Part model, mm, in its own coordinate system. A direction names the side the tool comes from. Give positions to 0.01 mm unless a question says otherwise; leave off trailing zeros. Order: outer loops, then holes, each group sorted by start corner. A loop starts at its lowest first (then second) coordinate and runs counter-clockwise, first axis right, second up.
1. Mould opens along Z. For faces 3 (the flat face through (20, 3, -41)), 4 (the flat face through (39, 3, -2)), 5 (the flat face through (3, 3, -36)) say: +Z half, -Z half, draft (parallel to the pull), parting line (faces both ways), or undercut.
2. Drop flat-ended pins along their axis: pin 1 Ø1 at (x, z) = (5, -12.5) entering from -Y; pin 2 Ø3 at (y, z) = (-5.5, -36.5) entering from -X; pin 3 Ø3.5 at (x, z) = (21, -6) entering from -Y. Give the stop position or say it passes through.
3. Which spindle directions (+Z, -Z, +X, -X, +Y, -Y) get a long thin tool onto all of the face, cutting with end or side? Do faces 1 (the cylindrical face through (32, -20.54, -10.57)), 2 (the cylindrical face through (37.2, 4, -4.1)). Say none if no direction does.
4. Probe line 1 (Z direction, x = 5, y = 1.85); line 2 (X direction, y = -22, z = -19); line 3 (Z direction, x = 10.5, y = -21.2). List the from-to ranges inside material, lowest first.
5. Slice it at A-A on y = -20. Give the number of separate pieces and of enclosed holes in the cut face, and give its area (3 significant figures).
6. Slice it at B-B on y = -11.5. List the corners of the cut face in (x, z).
from build123d import *

# Parameters (mm, degrees)
SKETCH1_W           = 41
SKETCH1_H           = 41
BOSS_EXTRUDE1_DEPTH = 5
CUT_EXTRUDE2_DEPTH  = 5
SKETCH4_R           = 11.5
CUT_EXTRUDE3_DEPTH  = 2
SKETCH6_R           = 17.5
BOSS_EXTRUDE2_DEPTH = 23
FILLET1_R           = 0.2
FILLET2_R           = 0.5
SKETCH13_R          = 11
BOSS_EXTRUDE3_DEPTH = 2
SKETCH5_R           = 3
CUT_EXTRUDE9_DEPTH  = 31
SKETCH14_R          = 2.5
CUT_EXTRUDE10_DEPTH = 5
SKETCH15_R          = 1.5
CUT_EXTRUDE11_DEPTH = 5
SKETCH16_R          = 2.5
CUT_EXTRUDE12_DEPTH = 3
SKETCH17_R          = 1.5
CUT_EXTRUDE13_DEPTH = 3
SKETCH18_R          = 1.5
CUT_EXTRUDE14_DEPTH = 5


with BuildPart() as part:
    # Sketch1 → Boss-Extrude1 (new body)
    with BuildSketch(Plane(origin=(0, 0, 0), x_dir=(1, 0, 0), z_dir=(0, 1, 0))):
        with Locations((20.5, 20.5)):
            Rectangle(SKETCH1_W, SKETCH1_H)
    extrude(amount=BOSS_EXTRUDE1_DEPTH)

    # Sketch2 → Cut-Extrude2 (cut)
    with BuildSketch(Plane(origin=(0, 5, 0), x_dir=(1, 0, 0), z_dir=(0, 1, 0))):
        Polygon((0, 4), (0, 0), (4, 0), align=None)
        Polygon((0, 41), (0, 37), (4, 41), align=None)
        Polygon((41, 41), (37, 41), (41, 37), align=None)
        Polygon((41, 4), (37, 0), (41, 0), align=None)
    extrude(amount=-CUT_EXTRUDE2_DEPTH, mode=Mode.SUBTRACT)

    # Sketch4 → Cut-Extrude3 (cut)
    with BuildSketch(Plane(origin=(0, 5, 0), x_dir=(1, 0, 0), z_dir=(0, 1, 0))):
        with Locations((20.5, 20.5)):
            Circle(SKETCH4_R)
    extrude(amount=-CUT_EXTRUDE3_DEPTH, mode=Mode.SUBTRACT)

    # Sketch6 → Boss-Extrude2 (add)
    with BuildSketch(Plane.XZ):
        with Locations((20.5, -20.5)):
            Circle(SKETCH6_R)
    extrude(amount=BOSS_EXTRUDE2_DEPTH)

    # Fillet1
    fillet1_edges = [part.edges().sort_by_distance(p)[0] for p in [
        (20.5, 0, 0),
        (2, 0, -2),
        (0, 0, -20.5),
        (2, 0, -39),
        (20.5, 0, -41),
        (39, 0, -39),
        (41, 0, -20.5),
        (39, 0, -2),
    ]]
    fillet(fillet1_edges, radius=FILLET1_R)

    # Fillet2
    fillet2_edges = [part.edges().sort_by_distance(p)[0] for p in [
        (3, -23, -20.5),
    ]]
    fillet(fillet2_edges, radius=FILLET2_R)

    # Sketch13 → Boss-Extrude3 (add)
    with BuildSketch(Plane(origin=(0, -23, 0), x_dir=(-1, 0, 0), z_dir=(0, -1, 0))):
        with Locations((-20.5, 20.5)):
            Circle(SKETCH13_R)
    extrude(amount=BOSS_EXTRUDE3_DEPTH)

    # Sketch5 → Cut-Extrude9 (cut, through all)
    with BuildSketch(Plane(origin=(0, 5, 0), x_dir=(1, 0, 0), z_dir=(0, 1, 0))):
        with Locations((20.5, 20.5)):
            Circle(SKETCH5_R)
    extrude(amount=-CUT_EXTRUDE9_DEPTH, mode=Mode.SUBTRACT)

    # Sketch14 → Cut-Extrude10 (cut)
    with BuildSketch(Plane(origin=(0, -23, 0), x_dir=(-1, 0, 0), z_dir=(0, -1, 0))):
        with Locations((-20.5, 6.5)):
            Circle(SKETCH14_R)
        with Locations((-34.5, 20.5)):
            Circle(SKETCH14_R)
        with Locations((-20.5, 34.5)):
            Circle(SKETCH14_R)
        with Locations((-6.5, 20.5)):
            Circle(SKETCH14_R)
    extrude(amount=-CUT_EXTRUDE10_DEPTH, mode=Mode.SUBTRACT)

    # Sketch15 → Cut-Extrude11 (cut)
    with BuildSketch(Plane(origin=(0, -23, 0), x_dir=(-1, 0, 0), z_dir=(0, -1, 0))):
        with Locations((-6.357864376, 20.5)):
            Circle(SKETCH15_R)
        with Locations((-30.5, 10.5)):
            Circle(SKETCH15_R)
        with Locations((-20.5, 6.357864376)):
            Circle(SKETCH15_R)
        with Locations((-30.5, 30.5)):
            Circle(SKETCH15_R)
        with Locations((-34.642135624, 20.5)):
            Circle(SKETCH15_R)
        with Locations((-10.5, 30.5)):
            Circle(SKETCH15_R)
        with Locations((-20.5, 34.642135624)):
            Circle(SKETCH15_R)
        with Locations((-10.5, 10.5)):
            Circle(SKETCH15_R)
    extrude(amount=-CUT_EXTRUDE11_DEPTH, mode=Mode.SUBTRACT)

    # Sketch16 → Cut-Extrude12 (cut)
    with BuildSketch(Plane(origin=(0, 0, 0), x_dir=(-1, 0, 0), z_dir=(0, -1, 0))):
        with Locations((-5, 5)):
            Circle(SKETCH16_R)
        with Locations((-36, 5)):
            Circle(SKETCH16_R)
        with Locations((-5, 36)):
            Circle(SKETCH16_R)
        with Locations((-36, 36)):
            Circle(SKETCH16_R)
    extrude(amount=-CUT_EXTRUDE12_DEPTH, mode=Mode.SUBTRACT)

    # Sketch17 → Cut-Extrude13 (cut, through all)
    with BuildSketch(Plane(origin=(0, 3, 0), x_dir=(-1, 0, 0), z_dir=(0, -1, 0))):
        with Locations((-5, 5)):
            Circle(SKETCH17_R)
        with Locations((-36, 5)):
            Circle(SKETCH17_R)
        with Locations((-5, 36)):
            Circle(SKETCH17_R)
        with Locations((-36, 36)):
            Circle(SKETCH17_R)
    extrude(amount=-CUT_EXTRUDE13_DEPTH, mode=Mode.SUBTRACT)

    # Sketch18 → Cut-Extrude14 (cut)
    with BuildSketch(Plane.XZ.offset(18)):
        with Locations((6.5, -20.5)):
            Circle(SKETCH18_R)
        with Locations((34.5, -20.5)):
            Circle(SKETCH18_R)
        with Locations((20.5, -6.5)):
            Circle(SKETCH18_R)
        with Locations((20.5, -34.5)):
            Circle(SKETCH18_R)
    extrude(amount=-CUT_EXTRUDE14_DEPTH, mode=Mode.SUBTRACT)


solid = part.part
Data:
1. face 3: -Z half
1. face 4: +Z half
1. face 5: undercut
2. pin 1: stops at y = -23
2. pin 2: stops at x = 10.7
2. pin 3: stops at y = -18
3. face 1: -Y
3. face 2: +Y, -Y
4. line 1: z = -41 to -38.5, -33.5 to -7.5, -2.5 to 0
4. line 2: x = 3.06 to 4.5, 8.5 to 17.9, 23.1 to 32.5, 36.5 to 37.94
4. line 3: z = -34.86 to -32, -29 to -12, -9 to -6.14
5. separate pieces: 1
5. enclosed holes: 9
5. area: 827 mm2
6. outline: circle Ø35 at (20.5, -20.5); hole circle Ø6 at (20.5, -20.5)
